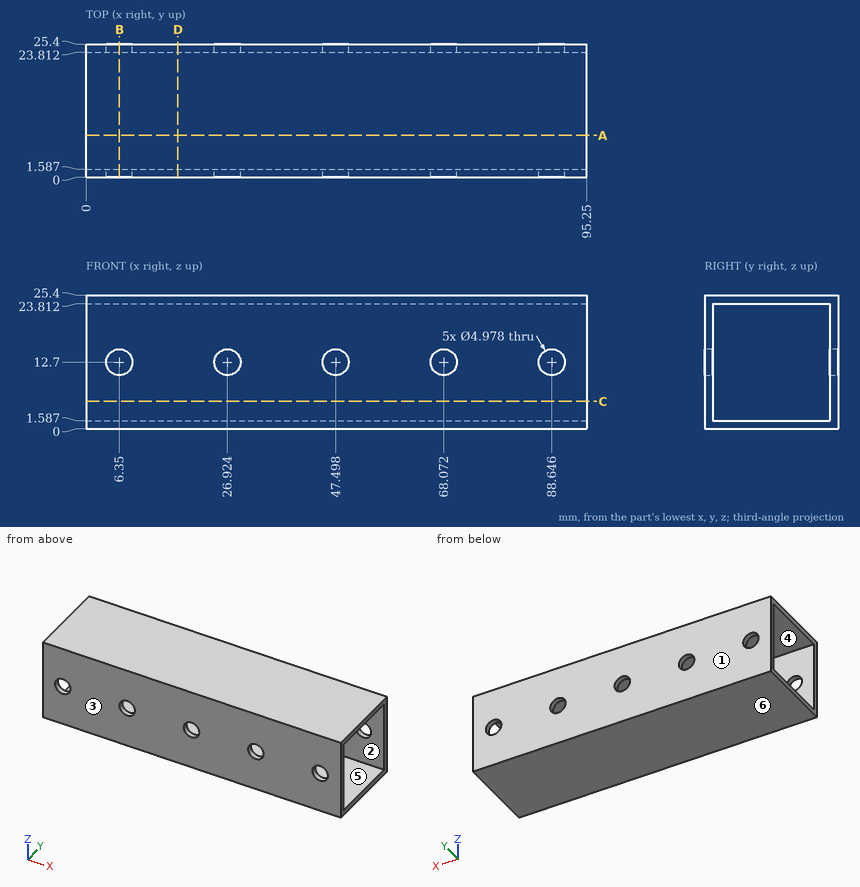
Design review of the part shown in the three views and the two pictorial views. Dimensions are in mm from the part's minimum x, y and z. A direction names the side the tool comes from. Round coordinates to 2 decimals unless told otherwise and drop trailing zeros. Write each loop counter-clockwise with the first axis right and the second up, starting at its lowest first coordinate (ties: lowest second). Pieces come first, ordered by that corner, then holes. Notation, with made-up numbers: (9.5, 15) - (66.5, 15) arc R18 ccw to (66.5, 20) - close; hole circle Ø10 at (-15, 58). An arc over 180 degrees is marked (long way). Answer as CSV lines item,"result". Start each with the question number.
(1) For line 1 (Z direction, x = 33, y = 21.5), list the stretches that pass through material, from the lowest coordinate up.
(2) Machinability: for the marked faces 1 and 2, which of the approach directions +Z, -Z, +X, -X, +Y, -Y give a long, thin tool a straight path to every point of the face, cutting with its end or side? Answer none if there is none.
(3) Add section B-B, the plane x = 6.35. State the section outline as (y, z) points.
(4) Add section D-D, the plane x = 17.5. State the section outline as (y, z) points, plus the area to 3 significant figures.
(5) Mouldability with a two-part tool opening along Y and no side actions: class the marked faces 3, 4, 5 and 6 as +Y half, -Y half, draft (parallel to the pull), parting line (faces both ways), or undercut.
(6) Add section A-A, the plane y = 8. State the section outline as (x, z) points.
(7) For pin 1 (8 mm diameter, centred on x = 47.498, z = 12.7, fed in from -Y), flat-tipped, find the tip position at first contact; note if it passes through.
From the geometry:
1,line 1,"z = 0 to 1.59, 23.81 to 25.4"
2,face 1,"+Z, -Z, +X, -X, +Y"
2,face 2,"+X, -X"
3,outline,"(0, 0) - (25.4, 0) - (25.4, 10.21) - (23.81, 10.21) - (23.81, 1.59) - (1.59, 1.59) - (1.59, 10.21) - (0, 10.21) - close; (0, 15.19) - (1.59, 15.19) - (1.59, 23.81) - (23.81, 23.81) - (23.81, 15.19) - (25.4, 15.19) - (25.4, 25.4) - (0, 25.4) - close"
4,outline,"(0, 0) - (25.4, 0) - (25.4, 25.4) - (0, 25.4) - close; hole (1.59, 1.59) - (23.81, 1.59) - (23.81, 23.81) - (1.59, 23.81) - close"
4,area,"151 mm²"
5,face 3,"-Y half"
5,face 4,"undercut"
5,face 5,"undercut"
5,face 6,"draft"
6,outline,"(0, 0) - (95.25, 0) - (95.25, 1.59) - (0, 1.59) - close; (0, 23.81) - (95.25, 23.81) - (95.25, 25.4) - (0, 25.4) - close"
7,pin 1,"stops at y = 0"
